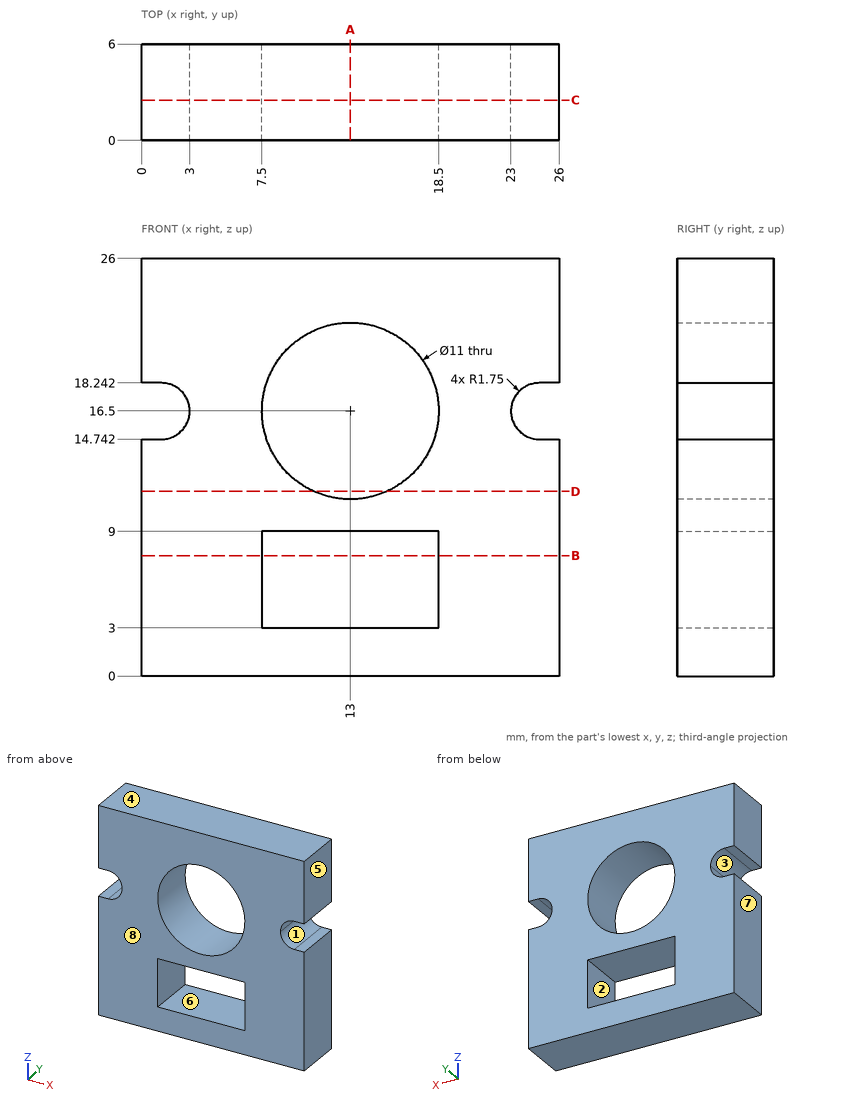
Drawing for the job (mm, zero at the part's lowest x, y, z). A direction names the side the tool comes from. Round coordinates to 2 decimals unless told otherwise and drop trailing zeros. Loops run counter-clockwise (first coordinate to the right, second up) from the corner with the lowest first, then second, coordinate; pieces in that order, holes last. Notation, with made-up numbers: (73, 19) - (119, 19) arc R30 ccw to (119, 57) - close; hole circle Ø3 at (7, 89.25). An arc over 180 degrees is marked (long way). Return JSON: item names as keys, results as strings. Group by question number.
Q1. Band-saw the part on A-A on x = 13. Give the cut face in (y, z), plus the area to 3 significant figures.
Q2. Flat gauge pin, fed straight in: pin 1 Ø1 at (y, z) = (3.5, 17) entering from +X. Where does the tip first touch, or does it go through?
Q3. Drill centre lines: line 1 along Z through (x, y) = (10.25, 5.5); line 2 along X through (y, z) = (0.75, 7.25); line 3 along X through (y, z) = (4.5, 16.5). Where is each one in solid material? Low to high. Write a range as [from, to].
Q4. Band-saw the part on B-B on z = 7.5. Give the cut face in (x, y).
Q5. Two-plate mould, pull along X, no slides. Class the marked faces 5, 6, 7 and 8: +X half, -X half, draft (parallel to the pull), parting line (faces both ways), or undercut.
Q6. Tool access for the marked faces 1, 2, 3 and 4: list every direction of +Z, -Z, +X, -X, +Y, -Y with a clear straight run to the whole face (end or side of a thin tool).
Q7. Band-saw the part on C-C on y = 2.5. Give the number of separate pieces and of enclosed holes in the cut face.
Q8. Band-saw the part on D-D on z = 11.5. Give the cut face in (x, y).
Solutions:
{
 "1": {"outline": "(0, 0) - (6, 0) - (6, 3) - (0, 3) - close; (0, 9) - (6, 9) - (6, 11) - (0, 11) - close; (0, 22) - (6, 22) - (6, 26) - (0, 26) - close", "area": "54.0 mm^2"},
 "2": {"pin 1": "stops at x = 23.32"},
 "3": {"line 1": "z = [0, 3], [9, 11.74], [21.26, 26]", "line 2": "x = [0, 7.5], [18.5, 26]", "line 3": "x = [3, 7.5], [18.5, 23]"},
 "4": {"outline": "(0, 0) - (7.5, 0) - (7.5, 6) - (0, 6) - close; (18.5, 0) - (26, 0) - (26, 6) - (18.5, 6) - close"},
 "5": {"face 5": "+X half", "face 6": "undercut", "face 7": "-X half", "face 8": "draft"},
 "6": {"face 1": "+X, +Y, -Y", "face 2": "+Y, -Y", "face 3": "-X, +Y, -Y", "face 4": "+Z, +X, -X, +Y, -Y"},
 "7": {"separate pieces": "1", "enclosed holes": "2"},
 "8": {"outline": "(0, 0) - (10.71, 0) - (10.71, 6) - (0, 6) - close; (15.29, 0) - (26, 0) - (26, 6) - (15.29, 6) - close"}
}
